from build123d import *

# Parameters (mm, degrees)
F1_DEPTH = 10
F2_R     = 2
F3_DEPTH = 5
F4_W     = 10
F4_H     = 2.5
F5_DEPTH = 3


with BuildPart() as f1:
    # F0 (on Top) → F1 (new body)
    with BuildSketch(Plane.XY):
        with BuildLine():
            ThreePointArc((0, -6), (4.242641, -4.242641), (6, 0))
            ThreePointArc((6, 0), (4.242641, 4.242641), (0, 6))
            Line((0, 6), (0, -6))
        make_face()
        with BuildLine():
            Line((0, -6), (0, 6))
            ThreePointArc((0, 6), (-6, 0), (0, -6))
        make_face()
    extrude(amount=F1_DEPTH)

    # F2 (on face) → F3 (cut)
    with BuildSketch(Plane.XY.offset(10)):
        Circle(F2_R)
    extrude(amount=-F3_DEPTH, mode=Mode.SUBTRACT)

    # F4 (on face) → F5 (cut)
    with BuildSketch(Plane(origin=(0, 0, 0), x_dir=(1, 0, 0), z_dir=(0, 0, -1))):
        Rectangle(F4_W, F4_H)
    extrude(amount=-F5_DEPTH, mode=Mode.SUBTRACT)


solid = f1.part
Input: part model. Units: mm. Frame: model coordinates. A direction names the side the tool comes from. Give positions to 0.01 mm unless a question says otherwise; leave off trailing zeros. Loops run counter-clockwise (first coordinate to the right, second up) from the corner with the lowest first, then second, coordinate; pieces in that order, holes last. Notation, with made-up numbers: M 23,82 L 42,82 A22 ccw 42,113 Z; hole C 34,-34.5 d10. An arc over 180 degrees is marked long. Use CSV: the item, a comma, the result in double quotes.
(1) Section D-D, the plane z = 8.75. Return loops of the section in (x, y), plus the area to 3 significant figures.
Outcome:
outline,"M 0,-6 A6 ccw 6,0 A6 ccw 0,6 A6 ccw Z; hole C 0,0 d4"
area,"101 mm²"
(2) Section A-A, the plane z = 2.5. Return loops of the section in (x, y), plus the area to 3 significant figures.
Outcome:
outline,"M 0,-6 A6 ccw 6,0 A6 ccw 0,6 A6 ccw Z; hole M -5,-1.25 L 5,-1.25 L 5,1.25 L -5,1.25 Z"
area,"88.1 mm²"
(3) Pin query (flat end, axial travel): P1, Ø4, axis at x = -2.5, z = 2.5, coming from the +Y side; P2, Ø1, axis at x = 5, z = 7, coming from the +Y side; P3, Ø2, axis at y = 3.5, z = 2.5, coming from the -X side. Return the tip coordinate at first contact, or that it passes through.
Outcome:
P1,"stops at y = 5.98"
P2,"stops at y = 3.97"
P3,"stops at x = -5.45"
(4) Pull-direction query (X, two-part tool) for faces 4 (the face through (-0.08, 1.42, 0)), 5 (the face through (0, 0, 5)); classes: pulls with the +X half, pulls with the -X half, needs draft (parallel to the pull), parting line crosses it, or undercut.
Outcome:
face 4,"needs draft"
face 5,"undercut"
(5) Set-up query: faces 1 (the face through (3, 0, 10)), 2 (the face through (0, -2, 8)), 3 (the face through (0, -1.25, 1)). Return all of +Z, -Z, +X, -X, +Y, -Y with unobstructed straight access to the full face (end or side cutting, diameter ignored); none if empty.
Outcome:
face 1,"+Z, +X, -X, +Y, -Y"
face 2,"+Z"
face 3,"-Z"
(6) Material intervals for L1, parallel to Y at x = 1.25, z = 1.5; L2, parallel to Y at x = 1.75, z = 6.5; L3, parallel to X at y = -1.5, z = 9.25, sorted ascending. Write a range as [from, to].
Outcome:
L1,"y = [-5.87, -1.25], [1.25, 5.87]"
L2,"y = [-5.74, -0.97], [0.97, 5.74]"
L3,"x = [-5.81, -1.32], [1.32, 5.81]"
(7) Section C-C, the plane y = -1.5. Return loops of the section in (x, z).
Outcome:
outline,"M -5.81,0 L 5.81,0 L 5.81,10 L 1.32,10 L 1.32,5 L -1.32,5 L -1.32,10 L -5.81,10 Z"
(8) Section B-B, the plane x = -0.5. Return loops of the section in (y, z).
Outcome:
outline,"M -5.98,0 L -1.25,0 L -1.25,3 L 1.25,3 L 1.25,0 L 5.98,0 L 5.98,10 L 1.94,10 L 1.94,5 L -1.94,5 L -1.94,10 L -5.98,10 Z"
